Here's the drawing with two shaded views (mm, measured from the low corner). I have some questions. Coordinates: 2 decimals unless noted, no trailing zeros. Write each loop counter-clockwise with the first axis right and the second up, starting at its lowest first coordinate (ties: lowest second). Pieces come first, ordered by that corner, then holes.
Item 1: I'm going to push flat-ended pins straight in: pin 1 Ø6 at (x, y) = (56, 9) entering from +Z; pin 2 Ø5 at (y, z) = (17, 15) entering from -X; pin 3 Ø6 at (x, y) = (49, 8.5) entering from +Z. Where does each tip first touch, or does it pass through?
Item 2: If we section it at C-C (y = 5.75): Please give me the cut outline in (x, z), then the cut area to 3 significant figures.
Item 3: If we section it at A-A (z = 36.83): Please give me the cut outline in (x, y), then the cut area to 3 significant figures.
Item 4: If I drill on line 1 (X direction, y = 5, z = 36.83); line 2 (Y direction, x = 38.5, z = 70.5), over which ranges is the centre line in solid material (lowest first)?
Item 5: If we section it at B-B (x = 36.83): Please give me the cut outline in (y, z).
Item 6: We'd pull the mould along Z, two halves only. Please class the marked faces 1, 2 and 3: +Z half, -Z half, draft (parallel to the pull), parting line (faces both ways), or undercut.
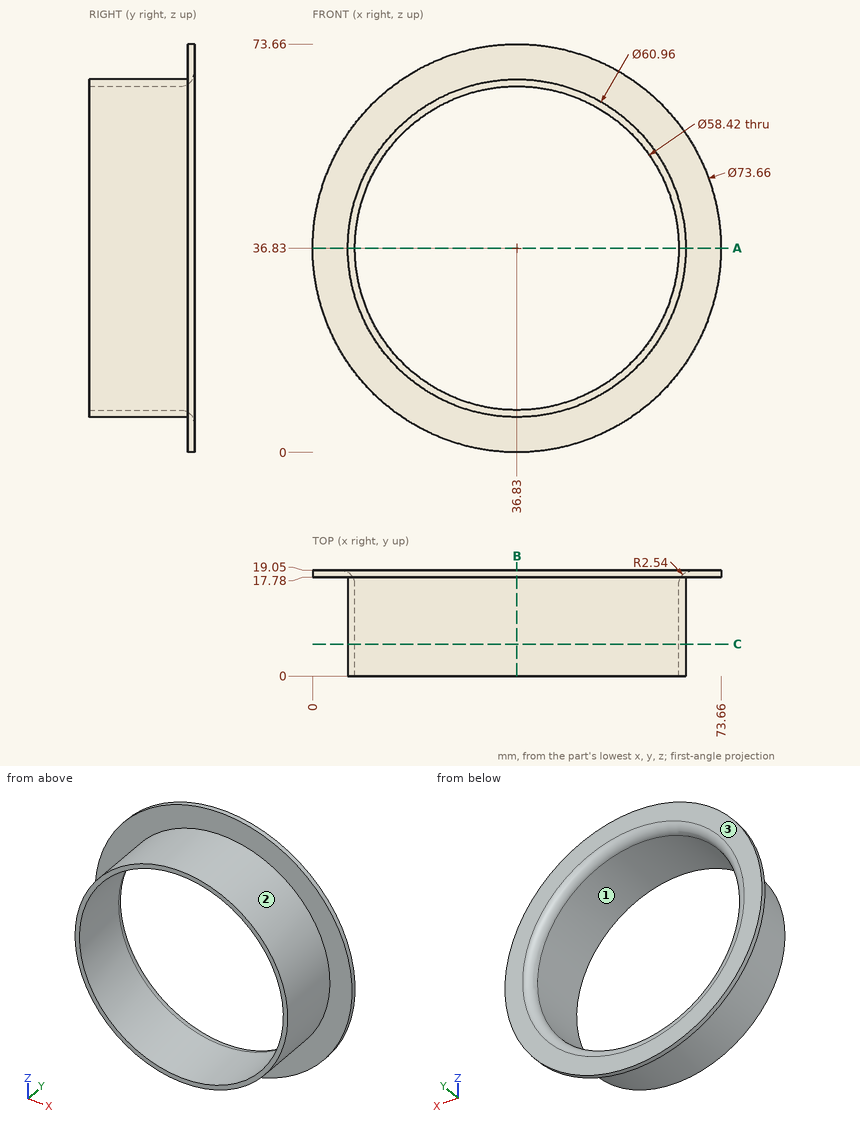
Answer list:
1. pin 1: stops at z = 62.67
1. pin 2: stops at x = 5.56
1. pin 3: stops at z = 65.9
2. outline: circle Ø60.96 at (36.83, 36.83); hole circle Ø58.42 at (36.83, 36.83)
2. area: 238 mm2
3. outline: (0, 17.78) - (6.35, 17.78) - (6.35, 0) - (7.62, 0) - (7.62, 16.51) arc R2.54 ccw to (5.08, 19.05) - (0, 19.05) - close; (66.04, 0) - (67.31, 0) - (67.31, 17.78) - (73.66, 17.78) - (73.66, 19.05) - (68.58, 19.05) arc R2.54 ccw to (66.04, 16.51) - close
3. area: 61.7 mm2
4. line 1: x = 6.35 to 7.62, 66.04 to 67.31
4. line 2: y = 17.78 to 19.05
5. outline: (0, 6.35) - (17.78, 6.35) - (17.78, 0) - (19.05, 0) - (19.05, 5.08) arc R2.54 ccw to (16.51, 7.62) - (0, 7.62) - close; (0, 66.04) - (16.51, 66.04) arc R2.54 ccw to (19.05, 68.58) - (19.05, 73.66) - (17.78, 73.66) - (17.78, 67.31) - (0, 67.31) - close
6. face 1: undercut
6. face 2: parting line
6. face 3: draft
